The listing builds one solid part. Answer for the finished solid, in the listing's coordinates (mm). A direction names the side the tool comes from. Round coordinates to 2 decimals unless told otherwise and drop trailing zeros. Write each loop counter-clockwise with the first axis right and the second up, starting at its lowest first coordinate (ties: lowest second). Pieces come first, ordered by that corner, then holes. Notation, with made-up numbers: (-40, 1.25) - (-30, 1.25) arc R13 cw to (-30, 21.25) - close; hole circle Ø4 at (72.25, 24.5). An arc over 180 degrees is marked (long way). Return JSON: item names as keys, results as strings. Group by question number.
(1) Section B-B, the plane x = 0 is taken. Write down the section's boundary in (y, z), then the cut area to 3 significant figures.
(2) Section D-D, the plane z = -11 is taken. Write down the section's boundary in (x, y), then the cut area to 3 significant figures.
(3) Find the intervals of material crossed by line 1 along Z through (x, y) = (-5.25, 0); line 2 along Y through (x, z) = (6, 32); line 3 along Z through (x, y) = (0, -8), in increasing order. Write a range as [from, to].
(4) Which of the six approach directions +Z, -Z, +X, -X, +Y, -Y give full straight-line access (tool end or side, diameter ignored) to faces 5 (the flat face through (12.5, 0, -32)), 6 (the flat face through (-8, -10, 19)), 7 (the flat face through (3.5, 5, 25.9))?
(5) Each of these flat-tipped pins is pushed along its axis until it touches: pin 1 (3.5 mm diameter, centred on y = 0, z = 34, fed in from -X); pin 2 (1.5 mm diameter, centred on y = -4.5, z = -23, fed in from -X); pin 3 (13 mm diameter, centred on x = 0, z = 22.5, fed in from +Y); pin 4 (5.5 mm diameter, centred on x = 0, z = 22.5, fed in from +Y). Where does it stop, or does it pass through?
(6) Section C-C, the plane x = -5.5 is taken. Write down the section's boundary in (y, z).
(7) Section A-A, the plane z = 22.5 is taken. Write down the section's boundary in (x, y), then the cut area to 3 significant figures.
(8) Determine the mould class of faces 1 (the flat face through (-1, 0, 32)), 2 (the cylindrical face through (0, 0, -21)), 3 (the flat face through (0.1, 13.4, -12.5)), 4 (the flat face through (8, 0, 37.5)) for opening direction Z: +Z half, -Z half, draft (parallel to the pull), parting line (faces both ways), or undercut.
Autodesk Inventor part; units mm, degrees
ref_plane "YZ Plane" through (0, 0, 0) normal (1, 0, 0) x (0, 1, 0)
ref_plane "XZ Plane" through (0, 0, 0) normal (0, 1, 0) x (-1, 0, 0)
ref_plane "XY Plane" through (0, 0, 0) normal (0, 0, 1) x (1, 0, 0)
sketch "Szkic1" plane through (0, 0, 0) normal (0, 0, 1) x (1, 0, 0)
  circle A0 centre (0, 0) radius 15
  dimension "d0" = 30
extrude "Wyciągnięcie proste1" add sketch "Szkic1" along normal mid plane 75
sketch "Szkic2" plane through (0, 0, -37.5) normal (0, 0, -1) x (-1, 0, 0)
  circle A0 centre (0, 0) radius 13
  circle A1 centre (0, 0) radius 15
  dimension "d3" = 26
  dimension "d4" = 30
extrude "Wyciągnięcie proste2" cut sketch "Szkic2" against normal blind 25
sketch "Szkic3" plane through (0, 0, 0) normal (1, 0, 0) x (0, 1, 0)
  circle A0 centre (0, -32.5) radius 1.5
  circle A1 centre (0, -22.5) radius 1.5
  line L0 (-13, -37.5) -> (13, -37.5)
  point P0 (0, 0)
  dimension "d7" = 3
  dimension "d8" = 3
  dimension "d13" = 10
  dimension "d14" = 5
extrude "Wyciągnięcie proste3" cut sketch "Szkic3" against normal blind 25 and the other way blind 12.5
thread "Gwint1"
thread "Gwint2"
sketch "Szkic4" plane through (0, 0, 0) normal (1, 0, 0) x (0, 1, 0)
  line L0 (15, 37.5) -> (-15, 37.5)
  line L1 (-15, 37.5) -> (-10, 37.5)
  line L2 (-10, 37.5) -> (-10, 7.5)
  line L3 (-15, 2.5) -> (-15, 2.5)
  line L4 (-15, 2.5) -> (-15, 37.5)
  line L5 (15, 37.5) -> (10, 37.5)
  line L6 (10, 37.5) -> (10, 7.5)
  line L7 (15, 2.5) -> (15, 2.5)
  line L8 (15, 2.5) -> (15, 37.5)
  arc A0 (-15, 2.5) -> (-10, 7.5) centre (-15, 7.5) ccw
  arc A1 (10, 7.5) -> (15, 2.5) centre (15, 7.5) ccw
  point P0 (0, 0)
  point P1 (-10, 2.5)
  point P2 (10, 2.5)
  dimension "d19" = 5
  dimension "d20" = 35
  dimension "d21" = 5
  dimension "d22" = 35
  dimension "d25" = 5
  dimension "d26" = 5
extrude "Wyciągnięcie proste4" cut sketch "Szkic4" along normal mid plane 30
sketch "Szkic6" plane through (-11.1803, 10, 7.5) normal (0, 1, 0) x (1, 0, 0)
  line L0 (-3.8197, -30) -> (0, -30) construction
  line L1 (0, 0) -> (22.3607, 0) construction
  line L2 (0, -30) -> (22.3607, -30) construction
  line L3 (22.3607, -30) -> (22.3607, 0) construction
  line L4 (22.3607, 0) -> (0, 0) construction
  line L5 (0, 0) -> (0, -30) construction
  circle A0 centre (11.1803, -15) radius 8.05
  point P0 (11.1803, 7.5)
  dimension "d30" = 16.1
extrude "Wyciągnięcie proste6" cut sketch "Szkic6" against normal blind 5
sketch "Szkic7" plane through (0, 5, 22.5) normal (0, 1, 0) x (1, 0, 0)
  circle A0 centre (0, 0) radius 4.5
  point P0 (0, 22.5)
  dimension "d33" = 9
extrude "Wyciągnięcie proste7" cut sketch "Szkic7" against normal blind 30
sketch "Szkic8" plane through (0, 0, 37.5) normal (0, 0, 1) x (1, 0, 0)
  line L0 (-1, 10) -> (1, 10)
  line L1 (1, 10) -> (1, -10)
  line L2 (1, -10) -> (-1, -10)
  line L3 (-1, -10) -> (-1, 10)
  line L4 (-1, 10) -> (1, -10) construction
  line L5 (1, 10) -> (-1, -10) construction
  point P0 (0, 0)
  dimension "d36" = 2
  dimension "d37" = 20
extrude "Wyciągnięcie proste8" cut sketch "Szkic8" against normal blind 12
sketch "Szkic9" plane through (1, -10, 37.5) normal (-1, 0, 0) x (0, 0, 1)
  circle A0 centre (-3.5, 10) radius 1.5
  point P0 (-37.5, 10)
  dimension "d40" = 3
extrude "Wyciągnięcie proste9" cut sketch "Szkic9" against normal blind 10 and the other way blind 20
thread "Gwint3"
sketch "Szkic10" plane through (-11.1803, -10, 7.5) normal (0, -1, 0) x (1, 0, 0)
  arc A0 (10.1803, 19.3875) -> (12.1803, 19.3875) centre (11.1803, 15) ccw
  circle A1 centre (11.1803, 15) radius 8.05
  point P0 (11.1803, -7.5)
  dimension "d49" = 16.1
extrude "Wyciągnięcie proste10" cut sketch "Szkic10" against normal blind 5
chamfer "Faza1" distance 2 angle 45 1 edges at (-15, -0.0202, 32.5001)
equation "\"d26\" = d25"
properties part number "koncowka" material "Aluminium 6061"
Working result:
{
 "1": {"outline": "(-15, -12.5) - (-13, -12.5) - (-13, -37.5) - (13, -37.5) - (13, -12.5) - (15, -12.5) - (15, 2.5) arc R5 cw to (10, 7.5) - (10, 14.45) - (5, 14.45) - (5, 18) - (-5, 18) - (-5, 14.45) - (-10, 14.45) - (-10, 7.5) arc R5 cw to (-15, 2.5) - close; hole circle Ø3 at (0, -32.5); hole circle Ø3 at (0, -22.5)", "area": "1,370 mm^2"},
 "2": {"outline": "circle Ø30 at (0, 0)", "area": "707 mm^2"},
 "3": {"line 1": "z = [-37.5, -34], [-31, -24], [-21, 32.5], [35.5, 37.5]", "line 2": "y = [-10, 10]", "line 3": "z = [-37.5, 14.45]"},
 "4": {"face 5": "-X", "face 6": "+Z, +X, -X, -Y", "face 7": "+Y"},
 "5": {"pin 1": "stops at x = -13.25", "pin 2": "stops at x = -12.45", "pin 3": "stops at y = 5", "pin 4": "passes through"},
 "6": {"outline": "(-13.96, -12.5) - (-11.78, -12.5) - (-11.78, -37.5) - (11.78, -37.5) - (11.78, -12.5) - (13.96, -12.5) - (13.96, 2.61) arc R5 cw to (10, 7.5) - (10, 16.62) - (5, 16.62) - (5, 28.38) - (10, 28.38) - (10, 37.5) - (-10, 37.5) - (-10, 28.38) - (-5, 28.38) - (-5, 16.62) - (-10, 16.62) - (-10, 7.5) arc R5 cw to (-13.96, 2.61) - close; hole circle Ø3 at (0, -32.5); hole circle Ø3 at (0, -22.5); hole circle Ø3 at (0, 34)"},
 "7": {"outline": "(-11.18, -10) - (-8.05, -10) - (-8.05, -5) - (-4.5, -5) - (-4.5, 5) - (-8.05, 5) - (-8.05, 10) - (-11.18, 10) arc R15 ccw to start; (4.5, -5) - (8.05, -5) - (8.05, -10) - (11.18, -10) arc R15 ccw to (11.18, 10) - (8.05, 10) - (8.05, 5) - (4.5, 5) - close", "area": "301 mm^2"},
 "8": {"face 1": "draft", "face 2": "undercut", "face 3": "-Z half", "face 4": "+Z half"}
}
